Read the model definition and answer for the solid it produces. Units are mm, in the model's axes. Coordinates: 2 decimals unless noted, no trailing zeros. Order: outer loops, then holes, each group sorted by start corner. A loop starts at its lowest first (then second) coordinate and runs counter-clockwise, first axis right, second up. Notation, with made-up numbers: M 9.5,25.25 L 22.5,25.25 A31 cw 22.5,57.25 Z; hole C 78,72 d10. An arc over 180 degrees is marked long. Write each question's results on one line, items separated by ' | '.
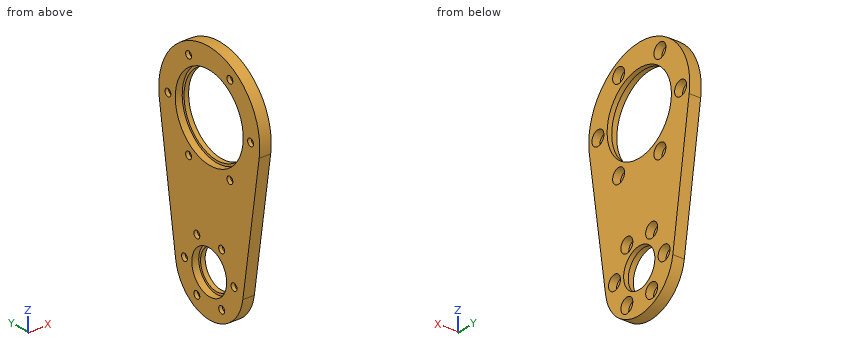
```python
from build123d import *

# Parameters (mm, degrees)
SKETCH_3_R                   = 27.5
EXTRUDE_1_DEPTH              = 2
SKETCH_4_R                   = 27.5
SKETCH_4_R_2                 = 17.5
EXTRUDE_2_DEPTH              = 1
SKETCH_5_R                   = 27.5
SKETCH_5_R_2                 = 18.5
EXTRUDE_3_DEPTH              = 7
SKETCH_6_R                   = 27.5
SKETCH_6_R_2                 = 17.5
EXTRUDE_4_DEPTH              = 2
EXTRUDE_5_DEPTH              = 9
SKETCH_11_R                  = 8.5
CUT_EXTRUDE_3_DEPTH          = 111
SKETCH_12_R                  = 9.5
CUT_EXTRUDE_4_DEPTH          = 2.5
SKETCH_13_R                  = 9.5
EXTRUDE_6_DEPTH              = 5
HOLE_WIZARD_M3_4_D           = 3.4
HOLE_WIZARD_M3_4_CBORE_D     = 6.5
HOLE_WIZARD_M3_4_CBORE_DEPTH = 3.4
PATTERN_CIRCULAR_1_COUNT     = 3
SKETCH_17_W                  = 25.034739103
SKETCH_17_H                  = 64.604217311
CUT_EXTRUDE_5_DEPTH          = 1111
HOLE_WIZARD_M3_2_D           = 3.2
HOLE_WIZARD_M3_2_CBORE_D     = 6.5
HOLE_WIZARD_M3_2_CBORE_DEPTH = 3.4
PATTERN_CIRCULAR_2_COUNT     = 6
HOLE_WIZARD_M3_3_D           = 3.2
HOLE_WIZARD_M3_3_CBORE_D     = 6.5
HOLE_WIZARD_M3_3_CBORE_DEPTH = 3.4
PATTERN_CIRCULAR_3_COUNT     = 6


with BuildPart() as part:
    # 스케치3 → 보스-돌출1 (new body)
    with BuildSketch(Plane(origin=(0, 0, 0), x_dir=(0, 0, -1), z_dir=(1, 0, 0))):
        Circle(SKETCH_3_R)
    extrude(amount=EXTRUDE_1_DEPTH)

    # 스케치4 → 보스-돌출2 (add)
    with BuildSketch(Plane(origin=(2, 0, 0), x_dir=(0, 0, -1), z_dir=(1, 0, 0))):
        Circle(SKETCH_4_R)
        Circle(SKETCH_4_R_2, mode=Mode.SUBTRACT)
    extrude(amount=EXTRUDE_2_DEPTH)

    # 스케치5 → 보스-돌출3 (add)
    with BuildSketch(Plane(origin=(3, 0, 0), x_dir=(0, 0, -1), z_dir=(1, 0, 0))):
        Circle(SKETCH_5_R)
        Circle(SKETCH_5_R_2, mode=Mode.SUBTRACT)
    extrude(amount=EXTRUDE_3_DEPTH)

    # 스케치6 → 보스-돌출4 (add)
    with BuildSketch(Plane(origin=(10, 0, 0), x_dir=(0, 0, -1), z_dir=(1, 0, 0))):
        Circle(SKETCH_6_R)
        Circle(SKETCH_6_R_2, mode=Mode.SUBTRACT)
    extrude(amount=EXTRUDE_4_DEPTH)

    # 스케치10 → 보스-돌출5 (add)
    with BuildSketch(Plane(origin=(12, 0, 0), x_dir=(0, 0, -1), z_dir=(1, 0, 0))):
        with BuildLine():
            Line((4.125, 27.188864908), (62.775, 18.290690938))
            ThreePointArc((62.775, 18.290690938), (78.5, 0), (62.775, -18.290690938))
            Line((62.775, -18.290690938), (4.125, -27.188864908))
            ThreePointArc((4.125, -27.188864908), (27.5, 0), (4.125, 27.188864908))
        make_face()
    extrude(amount=-EXTRUDE_5_DEPTH)

    # 스케치11 → 컷-돌출3 (cut, symmetric)
    with BuildSketch(Plane(origin=(7.5, 0, 0), x_dir=(0, 0, -1), z_dir=(1, 0, 0))):
        with Locations((60, 0)):
            Circle(SKETCH_11_R)
    extrude(amount=CUT_EXTRUDE_3_DEPTH, both=True, mode=Mode.SUBTRACT)

    # 스케치12 → 컷-돌출4 (cut, symmetric)
    with BuildSketch(Plane(origin=(7.5, 0, 0), x_dir=(0, 0, -1), z_dir=(1, 0, 0))):
        with Locations((60, 0)):
            Circle(SKETCH_12_R)
    extrude(amount=CUT_EXTRUDE_4_DEPTH, both=True, mode=Mode.SUBTRACT)

    # 스케치13 → 보스-돌출6 (add)
    with BuildSketch(Plane.ZY):
        Circle(SKETCH_13_R)
    extrude(amount=EXTRUDE_6_DEPTH)

    # M3 육각 소켓 머리 캡 나사용 카운터보어4 (through all)
    with Locations(Plane(origin=(2, 0, 0), x_dir=(0, 0, -1), z_dir=(1, 0, 0))):
        with Locations((0, 5)):
            hole_wizard_m3_4 = CounterBoreHole(HOLE_WIZARD_M3_4_D / 2, HOLE_WIZARD_M3_4_CBORE_D / 2, HOLE_WIZARD_M3_4_CBORE_DEPTH)

    # 원형 패턴1: M3 육각 소켓 머리 캡 나사용 카운터보어4 ×3 about axis
    pattern_circular_1_axis = Axis((0, 0, 0), (1, 0, 0))
    for i in range(1, PATTERN_CIRCULAR_1_COUNT):
        add(hole_wizard_m3_4.rotate(pattern_circular_1_axis, i * 360 / PATTERN_CIRCULAR_1_COUNT), mode=Mode.SUBTRACT)

    # 스케치17 → 컷-돌출5 (cut, symmetric)
    with BuildSketch(Plane.XY):
        with Locations((-5.517369551, -1.852450676)):
            Rectangle(SKETCH_17_W, SKETCH_17_H)
    extrude(amount=CUT_EXTRUDE_5_DEPTH, both=True, mode=Mode.SUBTRACT)

    # M3 육각 소켓 머리 캡 나사용 카운터보어2 (through all)
    with Locations(Plane(origin=(12, 0, 0), x_dir=(0, 0, -1), z_dir=(1, 0, 0))):
        with Locations((0, 22.5)):
            hole_wizard_m3_2 = CounterBoreHole(HOLE_WIZARD_M3_2_D / 2, HOLE_WIZARD_M3_2_CBORE_D / 2, HOLE_WIZARD_M3_2_CBORE_DEPTH)

    # 원형 패턴2: M3 육각 소켓 머리 캡 나사용 카운터보어2 ×6 about axis
    pattern_circular_2_axis = Axis((0, 0, 0), (1, 0, 0))
    for i in range(1, PATTERN_CIRCULAR_2_COUNT):
        add(hole_wizard_m3_2.rotate(pattern_circular_2_axis, i * 360 / PATTERN_CIRCULAR_2_COUNT), mode=Mode.SUBTRACT)

    # M3 육각 소켓 머리 캡 나사용 카운터보어3 (through all)
    with Locations(Plane(origin=(12, 0, 0), x_dir=(0, 0, -1), z_dir=(1, 0, 0))):
        with Locations((60, 13.5)):
            hole_wizard_m3_3 = CounterBoreHole(HOLE_WIZARD_M3_3_D / 2, HOLE_WIZARD_M3_3_CBORE_D / 2, HOLE_WIZARD_M3_3_CBORE_DEPTH)

    # 원형 패턴3: M3 육각 소켓 머리 캡 나사용 카운터보어3 ×6 about axis
    pattern_circular_3_axis = Axis((0, 0, -60), (1, 0, 0))
    for i in range(1, PATTERN_CIRCULAR_3_COUNT):
        add(hole_wizard_m3_3.rotate(pattern_circular_3_axis, i * 360 / PATTERN_CIRCULAR_3_COUNT), mode=Mode.SUBTRACT)


solid = part.part
```
(1) The part is cut by section B-B, the plane z = 6.5. Write down the section's boundary in (x, y).
Conclusion:
outline: M 7,-26.72 L 12,-26.72 L 12,-16.25 L 10,-16.25 L 10,-17.32 L 7,-17.32 Z; M 7,17.32 L 10,17.32 L 10,16.25 L 12,16.25 L 12,26.72 L 7,26.72 Z
(2) The part is cut by section C-C, the plane y = 22.5. Write down the section's boundary in (x, z).
Conclusion:
outline: M 7,-35.03 L 12,-35.03 L 12,-3.25 L 8.6,-3.25 L 8.6,-1.6 L 7,-1.6 Z; M 7,1.6 L 8.6,1.6 L 8.6,3.25 L 12,3.25 L 12,15.81 L 7,15.81 Z
(3) The part is cut by section A-A, the plane y = -1. Write down the section's boundary in (x, z).
Conclusion:
outline: M 7,-78.47 L 12,-78.47 L 12,-68.44 L 10,-68.44 L 10,-69.45 L 7,-69.45 Z; M 7,-50.55 L 10,-50.55 L 10,-51.56 L 12,-51.56 L 12,-17.47 L 10,-17.47 L 10,-18.47 L 7,-18.47 Z; M 7,18.47 L 10,18.47 L 10,17.47 L 12,17.47 L 12,27.48 L 7,27.48 Z
(4) Straight lines are drawn through the part: line 1 (Z direction, x = 11.3, y = 3); line 2 (Y direction, x = 7.65, z = -1); line 3 (Y direction, x = 9.65, z = -62). For each, find the intervals that lie inside material, in ascending order.
Conclusion:
line 1: -78.26 to -67.95, -52.05 to -17.24, 17.24 to 27.34 | line 2: -27.48 to -23.75, -21.25 to -18.47, 18.47 to 21.25, 23.75 to 27.48 | line 3: -18.41 to -16.06, -10.94 to -9.29, 9.29 to 10.94, 16.06 to 18.41
(5) The part is cut by section D-D, the plane x = 10.75. Count the separate pieces of the cut face and the enclosed holes in it, then the cut area to 3 significant figures.
Conclusion:
separate pieces: 1 | enclosed holes: 14 | area: 2,930 mm²
(6) Given pin 1 (6 mm diameter, centred on y = -11.25, z = -19.49, fed in from -X); pin 2 (5 mm diameter, centred on y = 22.5, z = 0, fed in from +X); pin 3 (1 mm diameter, centred on x = 9, z = -51.5, fed in from -Y); pin 4 (18.5 mm diameter, centred on y = 1.5, z = 8.5, fed in from -X), each flat-ended and moving along its own axis, determine where each tip first touches the part or whether it passes through.
Conclusion:
pin 1: x = 7 | pin 2: x = 8.6 | pin 3: y = -20.08 | pin 4: x = 10
